```python
from build123d import *

# Parameters (mm, degrees)
F0_W     = 101.6
F0_H     = 50.8
F0_W_2   = 88.9
F0_H_2   = 38.1
F1_DEPTH = 76.2
F2_W     = 88.9
F2_H     = 38.1
F3_DEPTH = 25.4
F4_R     = 6.35
F5_DEPTH = 25.4


with BuildPart() as f1:
    # F0 (on Front) → F1 (new body)
    with BuildSketch(Plane.XZ):
        with Locations((50.8, 25.4)):
            Rectangle(F0_W, F0_H)
        with Locations((50.8, 25.4)):
            Rectangle(F0_W_2, F0_H_2, mode=Mode.SUBTRACT)
    extrude(amount=F1_DEPTH)

    # F2 (on Front) → F3 (join)
    with BuildSketch(Plane.XZ):
        with Locations((50.8, 25.4)):
            Rectangle(F2_W, F2_H)
    extrude(amount=F3_DEPTH)

    # F4 (on face) → F5 (cut)
    with BuildSketch(Plane.XY.offset(50.8)):
        with Locations((25.4, -57.15)):
            Circle(F4_R)
        with Locations((76.2, -57.15)):
            Circle(F4_R)
    extrude(amount=-F5_DEPTH, mode=Mode.SUBTRACT)


solid = f1.part
```
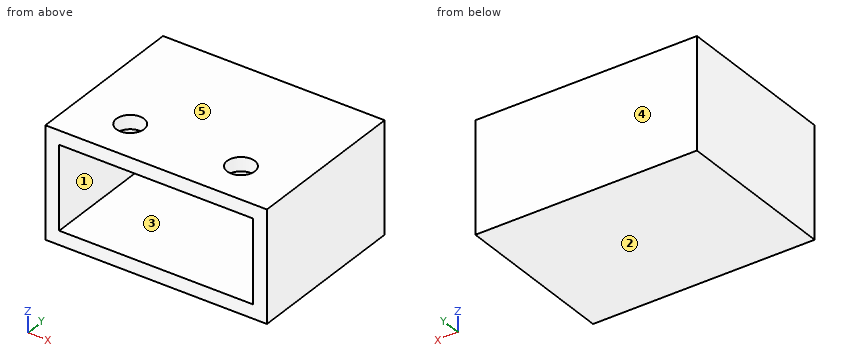
Build history of the part. All positions in model axes, mm. Face numbers are marked on the shaded views. A direction names the side the tool comes from. Give positions to 0.01 mm unless a question says otherwise; leave off trailing zeros. Loops run counter-clockwise (first coordinate to the right, second up) from the corner with the lowest first, then second, coordinate; pieces in that order, holes last. Notation, with made-up numbers: (7.5, 63.5) - (48.5, 63.5) arc R15 ccw to (48.5, 72.5) - close; hole circle Ø10 at (74.25, -39.75). An arc over 180 degrees is marked (long way). Use a Markdown table: item, result.
(1) Wall check: line 1 along Y through (x, z) = (76.2, 47.75); line 2 along X through (y, z) = (-57, 46); line 3 along Z through (x, y) = (36.5, -55.5). Give the ranges that are in metal, low to high.
Taken from the geometry:
| item | result |
|---|---|
| line 1 | -76.2 to -63.5, -50.8 to 0 |
| line 2 | 0 to 19.05, 31.75 to 69.85, 82.55 to 101.6 |
| line 3 | 0 to 6.35, 44.45 to 50.8 |
(2) Band-saw the part on D-D (z = 19.5). Give the cut face in (x, y).
Taken from the geometry:
| item | result |
|---|---|
| outline | (0, -76.2) - (6.35, -76.2) - (6.35, -25.4) - (95.25, -25.4) - (95.25, -76.2) - (101.6, -76.2) - (101.6, 0) - (0, 0) - close |
(3) Band-saw the part on A-A (x = 25.4). Give the cut face in (y, z).
Taken from the geometry:
| item | result |
|---|---|
| outline | (-76.2, 0) - (0, 0) - (0, 50.8) - (-50.8, 50.8) - (-50.8, 44.45) - (-25.4, 44.45) - (-25.4, 6.35) - (-76.2, 6.35) - close; (-76.2, 44.45) - (-63.5, 44.45) - (-63.5, 50.8) - (-76.2, 50.8) - close |
(4) Which spindle directions (+Z, -Z, +X, -X, +Y, -Y) get a long thin tool onto all of the face, cutting with end or side? Do the marked faces 1 and 2. Say none if no direction does.
Taken from the geometry:
| item | result |
|---|---|
| face 1 | -Y |
| face 2 | -Z, +X, -X, +Y, -Y |
(5) Drop flat-ended pins along their axis: pin 1 Ø4 at (x, y) = (26, -16.5) entering from -Z; pin 2 Ø3 at (x, z) = (87, 37.5) entering from -Y; pin 3 Ø11.5 at (x, y) = (76.2, -57.15) entering from +Z. Give the stop position or say it passes through.
Taken from the geometry:
| item | result |
|---|---|
| pin 1 | z = 0 |
| pin 2 | y = -25.4 |
| pin 3 | z = 6.35 |
(6) Band-saw the part on B-B (y = -27.5). Give the cut face in (x, z), and give its area (3 significant figures).
Taken from the geometry:
| item | result |
|---|---|
| outline | (0, 0) - (101.6, 0) - (101.6, 50.8) - (0, 50.8) - close; hole (6.35, 6.35) - (95.25, 6.35) - (95.25, 44.45) - (6.35, 44.45) - close |
| area | 1,770 mm2 |
(7) Band-saw the part on C-C (y = -57.15). Give the cut face in (x, z), and give its area (3 significant figures).
Taken from the geometry:
| item | result |
|---|---|
| outline | (0, 0) - (101.6, 0) - (101.6, 50.8) - (82.55, 50.8) - (82.55, 44.45) - (95.25, 44.45) - (95.25, 6.35) - (6.35, 6.35) - (6.35, 44.45) - (19.05, 44.45) - (19.05, 50.8) - (0, 50.8) - close; (31.75, 44.45) - (69.85, 44.45) - (69.85, 50.8) - (31.75, 50.8) - close |
| area | 1,610 mm2 |
(8) Pull direction Z, two halves, no side cores. Call the marked faces 3, 4 and 5: +Z half, -Z half, draft (parallel to the pull), parting line (faces both ways), or undercut.
Taken from the geometry:
| item | result |
|---|---|
| face 3 | undercut |
| face 4 | draft |
| face 5 | +Z half |
